For this review, take the finished solid that the model builds, in its own axes (mm). A direction names the side the tool comes from. Coordinates: 2 decimals unless noted, no trailing zeros. Loops run counter-clockwise (first coordinate to the right, second up) from the corner with the lowest first, then second, coordinate; pieces in that order, holes last. Notation, with made-up numbers: (12, 81.25) -> (51, 81.25) arc R8 cw to (51, 96.25) -> close; hole circle Ø6 at (-32, -23.5). An arc over 180 degrees is marked (long way). Answer in a Markdown table with one row per item.
from build123d import *

# Parameters (mm, degrees)
SKETCH1_W               = 8
SKETCH1_H               = 8
BOSS_EXTRUDE1_DEPTH     = 3
CUT_EXTRUDE1_DEPTH      = 12.704699911
CUT_EXTRUDE1_DEPTH_BACK = 12.704699911
CUT_EXTRUDE2_DEPTH      = 11
SKETCH4_R               = 1.75
CUT_EXTRUDE3_DEPTH      = 0.4
SKETCH5_W               = 8
SKETCH5_H               = 1
BOSS_EXTRUDE2_DEPTH     = 2
FILLET1_R               = 4
CUT_EXTRUDE4_DEPTH      = 0.4


with BuildPart() as part:
    # Sketch1 → Boss-Extrude1 (new body)
    with BuildSketch(Plane(origin=(0, 0, 0), x_dir=(1, 0, 0), z_dir=(0, 1, 0))):
        with Locations((4, 4)):
            Rectangle(SKETCH1_W, SKETCH1_H)
    extrude(amount=BOSS_EXTRUDE1_DEPTH)

    # Sketch2 → Cut-Extrude1 (cut, two sides: drawn at the far end of the back side and taken through both)
    with BuildSketch(Plane.XY.offset(-CUT_EXTRUDE1_DEPTH_BACK)):
        Polygon((0, 0), (0.6, 3), (0, 3), align=None)
        Polygon((8, 0), (7.4, 3), (8, 3), align=None)
    extrude(amount=CUT_EXTRUDE1_DEPTH + CUT_EXTRUDE1_DEPTH_BACK, mode=Mode.SUBTRACT)

    # Sketch3 → Cut-Extrude2 (cut)
    with BuildSketch(Plane(origin=(0, 0, 0), x_dir=(0, 0, -1), z_dir=(1, 0, 0))):
        Polygon((0, 0), (0.6, 3), (0, 3), align=None)
        Polygon((8, 3), (7.4, 3), (8, 0), align=None)
    extrude(amount=CUT_EXTRUDE2_DEPTH, mode=Mode.SUBTRACT)

    # Sketch4 → Cut-Extrude3 (cut)
    with BuildSketch(Plane.XZ):
        with Locations(Location((4, -3.75, 0), (0, 0, 270))):
            Circle(SKETCH4_R)
    extrude(amount=-CUT_EXTRUDE3_DEPTH, mode=Mode.SUBTRACT)

    # Sketch5 → Boss-Extrude2 (add)
    with BuildSketch(Plane.XZ):
        with Locations((4, -7.5)):
            Rectangle(SKETCH5_W, SKETCH5_H)
    extrude(amount=BOSS_EXTRUDE2_DEPTH)

    # Fillet1
    # the kernel refuses this fillet: 4 mm, written as the material it takes off along each edge
    with BuildSketch(Plane(origin=(8, -2, -16.660254038), x_dir=(0, 1, 0), z_dir=(0, 0, 1)), Plane(origin=(0, -2, 1.660254038), x_dir=(0, 1, 0), z_dir=(0, 0, -1))) as fillet1_piece_1:
        with BuildLine():
            CenterArc((4, 3.464101615), FILLET1_R, 180, 60)
            Line((0, 3.464101615), (-0.08, 3.464101615))
            Line((-0.08, 3.464101615), (-0.08, 0))
            Line((-0.08, 0), (0, -0.08))
            ThreePointArc((0, -0.08), (1, -0.08), (1.96, -0.069282032))
            Line((1.96, -0.069282032), (2, 0))
        make_face()
    extrude(amount=18.320508076, mode=Mode.SUBTRACT)

    # Sketch6 → Cut-Extrude4 (cut)
    with BuildSketch(Plane(origin=(0, 3, 0), x_dir=(1, 0, 0), z_dir=(0, 1, 0))):
        Polygon((2.428562008, 1.972012859), (2.428562008, 5.972012859), (3.232247906, 5.972012859), (4.838818418, 3.342205167), (4.838818418, 5.972012859), (5.608049188, 5.972012859), (5.608049188, 1.972012859), (4.779523547, 1.972012859), (3.197792777, 4.560153885), (3.197792777, 1.972012859), align=None)
    extrude(amount=-CUT_EXTRUDE4_DEPTH, mode=Mode.SUBTRACT)


solid = part.part
Item 1: Take a section at A-A, the plane y = 0.1. State the section outline as (x, z) points, and give its area (3 significant figures).
Worked answers:
| item | result |
|---|---|
| outline | (0.02, -7.98) -> (7.98, -7.98) -> (7.98, -0.02) -> (0.02, -0.02) -> close; hole circle Ø3.5 at (4, -3.75) |
| area | 53.7 mm² |
Item 2: Take a section at B-B, the plane x = 1.25. State the section outline as (y, z) points, and give its area (3 significant figures).
Worked answers:
| item | result |
|---|---|
| outline | (-1.33, -8) -> (0, -8) -> (3, -7.4) -> (3, -0.6) -> (0, 0) -> (0, -7) -> (-1.33, -7) -> close |
| area | 23.5 mm² |
Item 3: The part is to be moulded in two halves that separate along Z. For faces 1 (the flat face through (4, -2, -7.5)), 2 (the flat face through (4, 2.6, -4)), 3 (the flat face through (4, -1, -7)), say which applies: +Z half, -Z half, draft (parallel to the pull), parting line (faces both ways), or undercut.
Worked answers:
| item | result |
|---|---|
| face 1 | draft |
| face 2 | undercut |
| face 3 | +Z half |
Item 4: Take a section at D-D, the plane y = 2.3. State the section outline as (x, z) points, and give its area (3 significant figures).
Worked answers:
| item | result |
|---|---|
| outline | (0.46, -7.54) -> (7.54, -7.54) -> (7.54, -0.46) -> (0.46, -0.46) -> close |
| area | 50.1 mm² |
Item 5: For faces 4 (the flat face through (7.7, 1.5, -4.1)), 5 (the cylindrical face through (2.94, 0.2, -2.36)), 6 (the flat face through (3, 0, -2)), 7 (the flat face through (4, 2.8, -3.25)), list the 3-axis set-ups (+Z, -Z, +X, -X, +Y, -Y) from which the entire face can be reached by the end or side of a thin tool; tool diameter is ignored.
Worked answers:
| item | result |
|---|---|
| face 4 | +Z, -Z, +X, +Y |
| face 5 | -Y |
| face 6 | +Z, +X, -X, -Y |
| face 7 | +Y |
Item 6: Take a section at C-C, the plane z = -3. State the section outline as (x, y) points, and give its area (3 significant figures).
Worked answers:
| item | result |
|---|---|
| outline | (0, 0) -> (2.42, 0) -> (2.42, 0.4) -> (5.58, 0.4) -> (5.58, 0) -> (8, 0) -> (7.4, 3) -> (5.61, 3) -> (5.61, 2.6) -> (4.15, 2.6) -> (4.15, 3) -> (3.2, 3) -> (3.2, 2.6) -> (2.43, 2.6) -> (2.43, 3) -> (0.6, 3) -> close |
| area | 20.0 mm² |
Item 7: Insertion check: pin 1 (1.5 mm diameter, centred on y = 2, z = -7, fed in from -X); pin 2 (4 mm diameter, centred on x = 4, z = -3.5, fed in from -Y). Each pin has a flat end and moves straight along its axis. Give the tip position at first contact, or say it passes through.
Worked answers:
| item | result |
|---|---|
| pin 1 | x = 0.25 |
| pin 2 | y = 0 |
Item 8: For L1, parallel to Y at x = 5.25, z = -1.5; L2, parallel to X at y = 0.25, z = -3.75; L3, parallel to Z at x = 7.75, y = -0.15, list the stretches that pass through material, from the lowest coordinate up.
Worked answers:
| item | result |
|---|---|
| L1 | 0 to 3 |
| L2 | 0.05 to 2.25, 5.75 to 7.95 |
| L3 | -8 to -7 |
